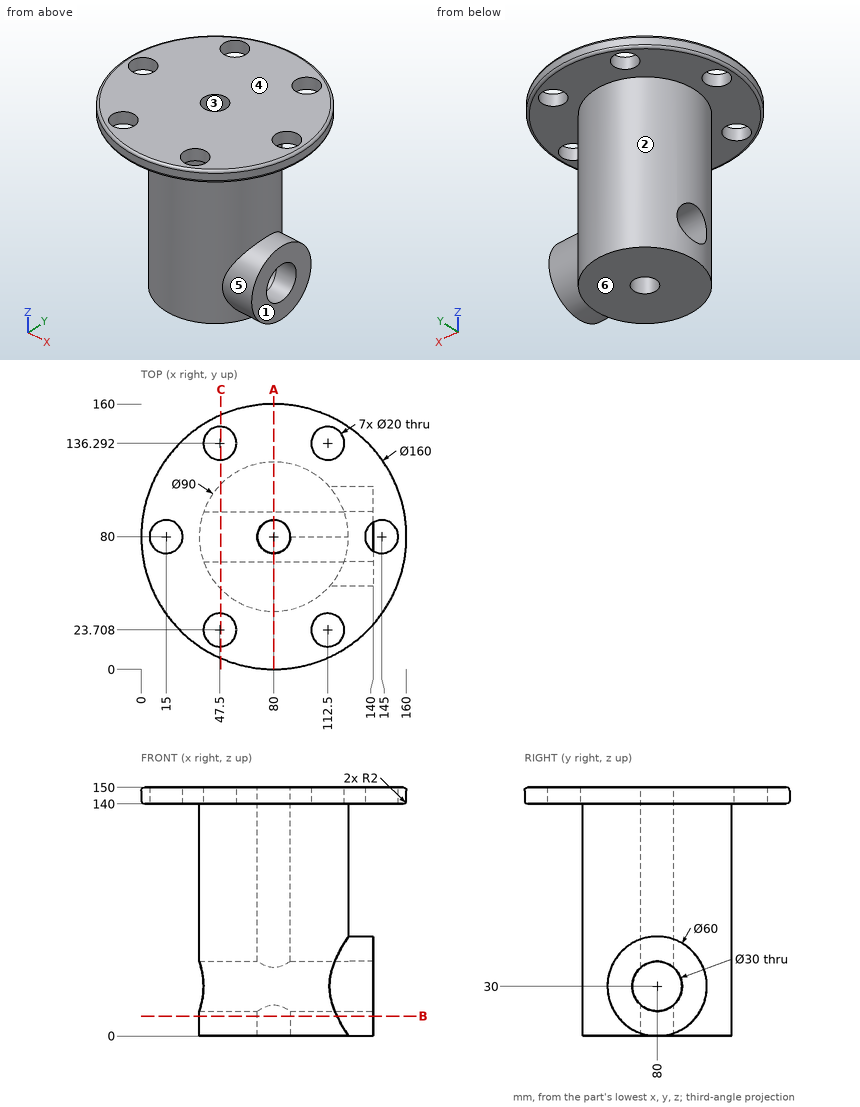
Check sheet for the drawn part. Datum: minimum x, y, z corner. Units: mm. A direction names the side the tool comes from. Give positions to 0.01 mm unless a question says otherwise; leave off trailing zeros. Order: outer loops, then holes, each group sorted by start corner. A loop starts at its lowest first (then second) coordinate and runs counter-clockwise, first axis right, second up.
1. Access from +Z, -Z, +X, -X, +Y, -Y to the whole of each face (thin tool, end or side, straight path). Record for the marked faces 5 and 6.
Completed:
face 5: +X
face 6: -Z, +X, -X, +Y, -Y
2. Sectioned sample at B-B (z = 12). Record the boundary of the cut face in (x, y).
Completed:
outline: (118.07, 56) - (140, 56) - (140, 104) - (118.07, 104) arc R45 ccw (long way) to start; hole circle Ø20 at (80, 80)
3. Draft check along X on the marked faces 1, 2, 3 and 4. Enter one of: pulls with the +X half, pulls with the -X half, needs draft (parallel to the pull), parting line crosses it, or undercut.
Completed:
face 1: pulls with the +X half
face 2: parting line crosses it
face 3: undercut
face 4: needs draft
4. Sectioned sample at C-C (x = 48). State how many separate pieces and enclosed holes the cut face has.
Completed:
separate pieces: 3
enclosed holes: 1
5. Scan lines: line 1 (Y direction, x = 131.5, z = 30); line 2 (Z direction, x = 122, y = 121); line 3 (Z direction, x = 120, y = 78). Record each from-to range of solid material in increasing order.
Completed:
line 1: y = 50 to 65, 95 to 110
line 2: z = 140 to 150
line 3: z = 0 to 15.13, 44.87 to 150
6. Sectioned sample at A-A (x = 80). Record the boundary of the cut face in (y, z).
Completed:
outline: (0, 142) arc R2 ccw to (2, 140) - (35, 140) - (35, 0) - (70, 0) - (70, 18.82) arc R15 cw to (70, 41.18) - (70, 150) - (2, 150) arc R2 ccw to (0, 148) - close; (90, 0) - (125, 0) - (125, 140) - (158, 140) arc R2 ccw to (160, 142) - (160, 148) arc R2 ccw to (158, 150) - (90, 150) - (90, 41.18) arc R15 cw to (90, 18.82) - close
7. Depth check by flat-ended pin: pin 1 (18 mm diameter, centred on y = 77, z = 37.5, fed in from +X); pin 2 (8 mm diameter, centred on x = 84, y = 74.5, fed in from +Z); pin 3 (12 mm diameter, centred on x = 69, z = 114, fed in from -Y); pin 4 (23 mm diameter, centred on x = 112.5, y = 136.29, fed in from -Z). Enter the tip coordinate at first touch or a pass-through.
Completed:
pin 1: stops at x = 140
pin 2: stops at z = 150
pin 3: stops at y = 35.28
pin 4: stops at z = 140
